Here's how the part is built. I have some questions about the finished solid (model axes, mm). Coordinates: 2 decimals unless noted, no trailing zeros. Write each loop counter-clockwise with the first axis right and the second up, starting at its lowest first coordinate (ties: lowest second). Pieces come first, ordered by that corner, then holes.
```python
from build123d import *

# Parameters (mm, degrees)
F0_R     = 25
F1_DEPTH = 50
F2_R     = 15
F3_DEPTH = 50.001
F4_W     = 91.62021
F4_H     = 76.697219
F5_DEPTH = 25


with BuildPart() as f1:
    # F0 (on Top) → F1 (new body)
    with BuildSketch(Plane.XY):
        Circle(F0_R)
    extrude(amount=F1_DEPTH)

    # F2 (on face) → F3 (cut, through all)
    with BuildSketch(Plane.XY.offset(50)):
        Circle(F2_R)
    extrude(amount=-F3_DEPTH, mode=Mode.SUBTRACT)

    # F4 (on Top) → F5 (join)
    with BuildSketch(Plane.XY):
        with Locations((9.023199, -1.041138)):
            Rectangle(F4_W, F4_H)
    extrude(amount=F5_DEPTH)


solid = f1.part
```
1) Imagine slicing it at A-A on y = 0. Please give me the cut outline in (x, z).
Values follow:
outline: (-36.79, 0) - (54.83, 0) - (54.83, 25) - (25, 25) - (25, 50) - (15, 50) - (15, 25) - (-15, 25) - (-15, 50) - (-25, 50) - (-25, 25) - (-36.79, 25) - close
2) Imagine slicing it at C-C on z = 45. Please give me the cut outline in (x, y), then the cut area to 3 significant figures.
Values follow:
outline: circle Ø50 at (0, 0); hole circle Ø30 at (0, 0)
area: 1,260 mm2
3) I need wall thicknesses on probe 1 along Y at (x, z) = (0, 33.75); probe 2 along Z at (x, y) = (6, -34); probe 3 along X at (y, z) = (-1, 32.5). Which ranges of each line are inside material? Lowest first, please.
Values follow:
probe 1: y = -25 to -15, 15 to 25
probe 2: z = 0 to 25
probe 3: x = -24.98 to -14.97, 14.97 to 24.98
4) Imagine slicing it at D-D on x = 40. Please give me the cut outline in (y, z).
Values follow:
outline: (-39.39, 0) - (37.31, 0) - (37.31, 25) - (-39.39, 25) - close
5) Will these pins go through, and if not, where does the flat tip stop? pin 1 (1.5 mm diameter, centred on x = -25, y = 18, fed in from +Z); pin 2 (1.5 mm diameter, centred on x = 17.5, z = 29.5, fed in from -Y); pin 3 (4 mm diameter, centred on x = 24.5, z = 44, fed in from +Y).
Values follow:
pin 1: stops at z = 25
pin 2: stops at y = -18.56
pin 3: stops at y = 10.9
6) Imagine slicing it at B-B on x = 0. Please give me the cut outline in (y, z), then the cut area to 3 significant figures.
Values follow:
outline: (-39.39, 0) - (37.31, 0) - (37.31, 25) - (25, 25) - (25, 50) - (15, 50) - (15, 25) - (-15, 25) - (-15, 50) - (-25, 50) - (-25, 25) - (-39.39, 25) - close
area: 2,420 mm2
7) We'd pull the mould along Y, two halves only. Please class faces 1 (the face through (8, 37.307, 12)), 2 (the face through (23.846, 7.509, 37.325)), 3 (the face through (-14.985, 0.66, 37.675)), 4 (the face through (0, 0, 25)): pulls with the +Y half, pulls with the -Y half, needs draft (parallel to the pull), parting line crosses it, or undercut.
Values follow:
face 1: pulls with the +Y half
face 2: parting line crosses it
face 3: undercut
face 4: undercut
